CAD build for the part. Positions are in the model's coordinates, mm. A direction names the side the tool comes from. Coordinates: 2 decimals unless noted, no trailing zeros. Order: outer loops, then holes, each group sorted by start corner. A loop starts at its lowest first (then second) coordinate and runs counter-clockwise, first axis right, second up. Notation, with made-up numbers: M 0.25,29 L 40.25,29 A24 ccw 40.25,60 Z; hole C -11.5,42.5 d11. An arc over 180 degrees is marked long. Write item = value, one per line.
from build123d import *

# Parameters (mm, degrees)
SKETCH1_W           = 20
SKETCH1_H           = 20
BOSS_EXTRUDE1_DEPTH = 20
SKETCH2_W           = 10
SKETCH2_H           = 10
CUT_EXTRUDE1_DEPTH  = 15
SKETCH3_W           = 20
SKETCH3_H           = 5
BOSS_EXTRUDE2_DEPTH = 2
LPATTERN1_COUNT     = 6
LPATTERN1_PITCH     = 22
SKETCH4_W           = 20
SKETCH4_H           = 15
BOSS_EXTRUDE3_DEPTH = 2
SKETCH5_W           = 20
SKETCH5_H           = 20
BOSS_EXTRUDE5_DEPTH = 2
SKETCH7_W           = 120
SKETCH7_H           = 2
CUT_EXTRUDE2_DEPTH  = 2
SKETCH8_W           = 134
SKETCH8_H           = 20
BOSS_EXTRUDE6_DEPTH = 6


with BuildPart() as part:
    # Sketch1 → Boss-Extrude1 (new body)
    with BuildSketch(Plane.XY):
        with Locations((10, 10)):
            Rectangle(SKETCH1_W, SKETCH1_H)
    extrude(amount=BOSS_EXTRUDE1_DEPTH)

    # Sketch2 → Cut-Extrude1 (cut)
    with BuildSketch(Plane(origin=(0, 0, 0), x_dir=(-1, 0, 0), z_dir=(0, -1, 0))):
        with Locations((-10, -10)):
            Rectangle(SKETCH2_W, SKETCH2_H)
    extrude(amount=-CUT_EXTRUDE1_DEPTH, mode=Mode.SUBTRACT)

    # Sketch3 → Boss-Extrude2 (add)
    with BuildSketch(Plane(origin=(20, 0, 0), x_dir=(0, 0, -1), z_dir=(1, 0, 0))):
        with Locations((-10, 2.5)):
            Rectangle(SKETCH3_W, SKETCH3_H)
    extrude(amount=BOSS_EXTRUDE2_DEPTH)


with BuildPart() as lpattern1_1:
    # LPattern1: pattern copy
    add(part.part.moved(Location(Vector(1, 0, 0) * (1 * LPATTERN1_PITCH))))


with BuildPart() as lpattern1_2:
    # LPattern1: pattern copy
    add(part.part.moved(Location(Vector(1, 0, 0) * (2 * LPATTERN1_PITCH))))


with BuildPart() as lpattern1_3:
    # LPattern1: pattern copy
    add(part.part.moved(Location(Vector(1, 0, 0) * (3 * LPATTERN1_PITCH))))


with BuildPart() as lpattern1_4:
    # LPattern1: pattern copy
    add(part.part.moved(Location(Vector(1, 0, 0) * (4 * LPATTERN1_PITCH))))


with BuildPart() as lpattern1_5:
    # LPattern1: pattern copy
    add(part.part.moved(Location(Vector(1, 0, 0) * (5 * LPATTERN1_PITCH))))


with BuildPart() as lpattern1_1_1:
    add(lpattern1_1.part)

    # Combine1: union LPattern1_2, LPattern1_3, part, LPattern1_4, LPattern1_5
    add(lpattern1_2.part)
    add(lpattern1_3.part)
    add(part.part)
    add(lpattern1_4.part)
    add(lpattern1_5.part)

    # Sketch4 → Boss-Extrude3 (add)
    with BuildSketch(Plane(origin=(130, 0, 0), x_dir=(0, 0, -1), z_dir=(1, 0, 0))):
        with Locations((-10, 12.5)):
            Rectangle(SKETCH4_W, SKETCH4_H)
    extrude(amount=BOSS_EXTRUDE3_DEPTH)

    # Sketch5 → Boss-Extrude5 (add)
    with BuildSketch(Plane.ZY):
        with Locations((10, 10)):
            Rectangle(SKETCH5_W, SKETCH5_H)
    extrude(amount=BOSS_EXTRUDE5_DEPTH)

    # Sketch7 → Cut-Extrude2 (cut)
    with BuildSketch(Plane(origin=(0, 0, 0), x_dir=(-1, 0, 0), z_dir=(0, -1, 0))):
        with Locations((-65, -10)):
            Rectangle(SKETCH7_W, SKETCH7_H)
    extrude(amount=-CUT_EXTRUDE2_DEPTH, mode=Mode.SUBTRACT)

    # Sketch8 → Boss-Extrude6 (add)
    with BuildSketch(Plane.XZ):
        with Locations((65, 10)):
            Rectangle(SKETCH8_W, SKETCH8_H)
    extrude(amount=BOSS_EXTRUDE6_DEPTH)


solid = lpattern1_1_1.part
(1) Wall check: line 1 (X direction, y = 18, z = 6.25); line 2 (Z direction, x = 13, y = 9). Give the ranges that are in metal, low to high. Write a range as from..to.
Evaluation:
line_1 = -2..20, 22..42, 44..64, 66..86, 88..108, 110..132
line_2 = 0..5, 15..20
(2) Pull direction Z, two halves, no side cores. Call faces 1 (the face through (64, -6, 10)), 2 (the face through (54, 7, 5)): +Z half, -Z half, draft (parallel to the pull), parting line (faces both ways), or undercut.
Evaluation:
face_1 = draft
face_2 = undercut
(3) Pin check, flat tip, straight feed: pin 1 Ø2 at (x, y) = (85.5, 0.5) entering from -Z. Stop position of the tip, or through.
Evaluation:
pin_1 = 0
(4) Slice it at C-C, the plane z = 2. Write the cut outline in (x, y).
Evaluation:
outline = M -2,-6 L 132,-6 L 132,20 L 110,20 L 110,5 L 108,5 L 108,20 L 88,20 L 88,5 L 86,5 L 86,20 L 66,20 L 66,5 L 64,5 L 64,20 L 44,20 L 44,5 L 42,5 L 42,20 L 22,20 L 22,5 L 20,5 L 20,20 L -2,20 Z
(5) Tool access for faces 3 (the face through (98, 20, 10)), 4 (the face through (20, 12, 10)), 5 (the face through (93, 7, 10)): list every direction of +Z, -Z, +X, -X, +Y, -Y with a clear straight run to the whole face (end or side of a thin tool).
Evaluation:
face_3 = +Z, -Z, +X, -X, +Y
face_4 = +Z, -Z, +Y
face_5 = none
(6) Slice it at B-B, the plane x = 53.5. Write the cut outline in (y, z).
Evaluation:
outline = M -6,0 L 20,0 L 20,20 L -6,20 Z; hole M 0,5 L 15,5 L 15,15 L 0,15 Z
(7) Slice it at D-D, the plane y = 7.75. State how many separate pieces and enclosed holes the cut face has, then the cut area to 3 significant figures.
Evaluation:
separate_pieces = 6
enclosed_holes = 6
area = 1,880 mm²
(8) Slice it at A-A, the plane y = 18.75. Write the cut outline in (x, z), then the cut area to 3 significant figures.
Evaluation:
outline = M -2,0 L 20,0 L 20,20 L -2,20 Z; M 22,0 L 42,0 L 42,20 L 22,20 Z; M 44,0 L 64,0 L 64,20 L 44,20 Z; M 66,0 L 86,0 L 86,20 L 66,20 Z; M 88,0 L 108,0 L 108,20 L 88,20 Z; M 110,0 L 132,0 L 132,20 L 110,20 Z
area = 2,480 mm²
